CAD build for the part. Positions are in the model's coordinates, mm. A direction names the side the tool comes from. Coordinates: 2 decimals unless noted, no trailing zeros. Order: outer loops, then holes, each group sorted by start corner. A loop starts at its lowest first (then second) coordinate and runs counter-clockwise, first axis right, second up. Notation, with made-up numbers: (39, 56.5) - (93, 56.5) arc R11 ccw to (93, 71.5) - close; hole circle Ø10 at (-5.75, -16.75). An arc over 180 degrees is marked (long way). Use one line per item in the form item = value.
```python
from build123d import *

# Parameters (mm, degrees)
SKETCH_1_W          = 65
SKETCH_1_H          = 70
EXTRUDE_1_DEPTH     = 3
SKETCH_2_W          = 65
SKETCH_2_H          = 6
EXTRUDE_2_DEPTH     = 21
SKETCH_3_W          = 65
SKETCH_3_H          = 3
EXTRUDE_3_DEPTH     = 26
SKETCH_4_W          = 39
SKETCH_4_H          = 3
CUT_EXTRUDE_1_DEPTH = 55.865745233
SKETCH_5_R          = 2
CUT_EXTRUDE_2_DEPTH = 82.76337811
SKETCH_6_W          = 65
SKETCH_6_H          = 3
EXTRUDE_4_DEPTH     = 13.6
SKETCH_7_R          = 2.5
CUT_EXTRUDE_3_DEPTH = 64.199762658
SKETCH_8_W          = 15
SKETCH_8_H          = 9
CUT_EXTRUDE_4_DEPTH = 64.199762658


with BuildPart() as part:
    # 草图1 → 凸台-拉伸1 (new body)
    with BuildSketch(Plane.XY):
        Rectangle(SKETCH_1_W, SKETCH_1_H)
    extrude(amount=EXTRUDE_1_DEPTH)

    # 草图2 → 凸台-拉伸2 (add)
    with BuildSketch(Plane.XY.offset(3)):
        with Locations((0, 32)):
            Rectangle(SKETCH_2_W, SKETCH_2_H)
    extrude(amount=EXTRUDE_2_DEPTH)

    # 草图3 → 凸台-拉伸3 (add)
    with BuildSketch(Plane(origin=(0, 35, 0), x_dir=(1, 0, 0), z_dir=(0, 1, 0))):
        with Locations((0, -25.5)):
            Rectangle(SKETCH_3_W, SKETCH_3_H)
    extrude(amount=-EXTRUDE_3_DEPTH)

    # 草图4 → 切除-拉伸1 (cut, through all)
    with BuildSketch(Plane.XY.offset(27)):
        with Locations((0, 33.5)):
            Rectangle(SKETCH_4_W, SKETCH_4_H)
    extrude(amount=-CUT_EXTRUDE_1_DEPTH, mode=Mode.SUBTRACT)

    # 草图5 → 切除-拉伸2 (cut, through all)
    with BuildSketch(Plane(origin=(0, 35, 0), x_dir=(1, 0, 0), z_dir=(0, 1, 0))):
        with Locations(Location((-25, -13.5, 0), (0, 0, 270))):
            Circle(SKETCH_5_R)
        with Locations(Location((25, -13.5, 0), (0, 0, 270))):
            Circle(SKETCH_5_R)
    extrude(amount=-CUT_EXTRUDE_2_DEPTH, mode=Mode.SUBTRACT)

    # 草图6 → 凸台-拉伸4 (add)
    with BuildSketch(Plane.XZ.offset(35)):
        with Locations((0, 1.5)):
            Rectangle(SKETCH_6_W, SKETCH_6_H)
    extrude(amount=EXTRUDE_4_DEPTH)

    # 草图7 → 切除-拉伸3 (cut, through all)
    with BuildSketch(Plane.XY.offset(3)):
        with Locations((-22.5, -39)):
            Circle(SKETCH_7_R)
        with Locations((22.5, -39)):
            Circle(SKETCH_7_R)
    extrude(amount=-CUT_EXTRUDE_3_DEPTH, mode=Mode.SUBTRACT)

    # 草图8 → 切除-拉伸4 (cut, through all)
    with BuildSketch(Plane.XY.offset(3)):
        with Locations((-10, -24.1)):
            Rectangle(SKETCH_8_W, SKETCH_8_H)
    extrude(amount=-CUT_EXTRUDE_4_DEPTH, mode=Mode.SUBTRACT)


solid = part.part
```
Item 1: 3-axis set-ups, long thin cutter, end or side, ignore diameter. For faces 1 (the face through (0, 32, 14)), 2 (the face through (0, 29, 13)), 3 (the face through (27.4, 35, 13.3)), 4 (the face through (-2.5, -24, 2)): which of +Z, -Z, +X, -X, +Y, -Y reach the whole face in a straight line?
Derived:
face_1 = +Z, -Z, +Y
face_2 = +X, -X, -Y
face_3 = +Z, -Z, +X, -X, +Y
face_4 = +Z, -Z
Item 2: Cut at D-D, the plane y = -39. Write the cut outline in (x, z).
Derived:
outline = (-32.5, 0) - (-25, 0) - (-25, 3) - (-32.5, 3) - close; (-20, 0) - (20, 0) - (20, 3) - (-20, 3) - close; (25, 0) - (32.5, 0) - (32.5, 3) - (25, 3) - close
Item 3: Drill centre lines: line 1 (X direction, y = 30.4, z = 13.5); line 2 (Y direction, x = 22.5, z = 2); line 3 (X direction, y = 32.15, z = 13.5). Where is each one in solid material? Low to high. Write a range as [from, to].
Derived:
line_1 = [-32.5, -27], [-23, 23], [27, 32.5]
line_2 = [-48.6, -41.5], [-36.5, 35]
line_3 = [-32.5, -27], [-23, -19.5], [19.5, 23], [27, 32.5]
Item 4: Cut at C-C, the plane x = -5. Write the cut outline in (y, z), plus the area to 3 significant figures.
Derived:
outline = (-48.6, 0) - (-28.6, 0) - (-28.6, 3) - (-48.6, 3) - close; (-19.6, 0) - (32, 0) - (32, 27) - (9, 27) - (9, 24) - (29, 24) - (29, 3) - (-19.6, 3) - close
area = 347 mm²
Item 5: Cut at A-A, the plane z = 13.5. Write the cut outline in (x, y).
Derived:
outline = (-32.5, 29) - (-27, 29) - (-27, 35) - (-32.5, 35) - close; (-23, 29) - (23, 29) - (23, 35) - (19.5, 35) - (19.5, 32) - (-19.5, 32) - (-19.5, 35) - (-23, 35) - close; (27, 29) - (32.5, 29) - (32.5, 35) - (27, 35) - close
Item 6: Cut at B-B, the plane y = 13.5. Write the cut outline in (x, z), plus the area to 3 significant figures.
Derived:
outline = (-32.5, 0) - (32.5, 0) - (32.5, 3) - (-32.5, 3) - close; (-32.5, 24) - (32.5, 24) - (32.5, 27) - (-32.5, 27) - close
area = 390 mm²
Item 7: Two-plate mould, pull along X, no slides. Class faces 5 (the face through (0, -9, 3)), 6 (the face through (-32.5, 9, 2)), 7 (the face through (-10, -28.6, 2)), 8 (the face through (32.5, 9, 2)): +X half, -X half, draft (parallel to the pull), parting line (faces both ways), or undercut.
Derived:
face_5 = draft
face_6 = -X half
face_7 = undercut
face_8 = +X half
Item 8: Drop flat-ended pins along their axis: pin 1 (1.5 mm diameter, centred on x = -10, z = 1.5, fed in from +Y); pin 2 (3 mm diameter, centred on x = -0.5, y = -4.5, fed in from +Z); pin 3 (10 mm diameter, centred on x = 23.5, z = 22.5, fed in from -Y); pin 4 (3 mm diameter, centred on x = 25, z = 13.5, fed in from +Y). Give the stop position or say it passes through.
Derived:
pin_1 = 32
pin_2 = 3
pin_3 = 9
pin_4 = through
